```python
from build123d import *

# Parameters (mm, degrees)
BOSS_EXTRUDE1_DEPTH = 4
CUT_EXTRUDE4_REACH  = 6
SKETCH2_R           = 1.55
CUT_EXTRUDE5_DEPTH  = 5
FILLET1_R           = 0.5


with BuildPart() as part:
    # Sketch1 → Boss-Extrude1 (new body)
    with BuildSketch(Plane.XY):
        with BuildLine():
            Line((-10, 14), (-7.553754025, 14))
            Line((-7.553754025, 14), (-7.550510257, 12.5))
            ThreePointArc((-7.550510257, 12.5), (-6.759629651, 8.677124344), (-10, 6.5))
            Line((-10, 6.5), (-11.5, 6.5))
            Line((-11.5, 6.5), (-11.5, -6.5))
            Line((-11.5, -6.5), (-10, -6.5))
            ThreePointArc((-10, -6.5), (-6.774250172, -8.641862287), (-7.496564289, -12.445978258))
            Line((-7.496564289, -12.445978258), (-7.493203699, -14))
            Line((-7.493203699, -14), (-10, -14))
            ThreePointArc((-10, -14), (-12.474873734, -12.974873734), (-13.5, -10.5))
            Line((-13.5, -10.5), (-13.5, 10.5))
            ThreePointArc((-13.5, 10.5), (-12.474873734, 12.974873734), (-10, 14))
        make_face()
    extrude(amount=BOSS_EXTRUDE1_DEPTH)

    # Sketch2 → Cut-Extrude4 (cut, up to next)
    with BuildSketch(Plane.XY, mode=Mode.PRIVATE) as cut_extrude4_sk1:
        with Locations((-10, -10)):
            Circle(SKETCH2_R)
    cut_extrude4_tool1 = extrude(cut_extrude4_sk1.sketch, amount=CUT_EXTRUDE4_REACH, mode=Mode.PRIVATE) & part.part
    add(cut_extrude4_tool1.solids().sort_by_distance((-10, -10, 0))[0], mode=Mode.SUBTRACT)
    # Sketch2 → Cut-Extrude4 (cut, up to next)
    with BuildSketch(Plane.XY, mode=Mode.PRIVATE) as cut_extrude4_sk2:
        with Locations((-10, 10)):
            Circle(SKETCH2_R)
    cut_extrude4_tool2 = extrude(cut_extrude4_sk2.sketch, amount=CUT_EXTRUDE4_REACH, mode=Mode.PRIVATE) & part.part
    add(cut_extrude4_tool2.solids().sort_by_distance((-10, 10, 0))[0], mode=Mode.SUBTRACT)

    # Sketch3 → Cut-Extrude5 (cut, through all)
    with BuildSketch(Plane.XY.offset(4)):
        with BuildLine():
            Line((-9.034256252, 11.212369174), (-6.716684452, 11.212369174))
            ThreePointArc((-6.716684452, 11.212369174), (-6.5, 10), (-6.716684452, 8.787630826))
            Line((-6.716684452, 8.787630826), (-9.034256252, 8.787630826))
            ThreePointArc((-9.034256252, 8.787630826), (-8.45, 10), (-9.034256252, 11.212369174))
        make_face()
    cut_extrude5 = extrude(amount=-CUT_EXTRUDE5_DEPTH, mode=Mode.SUBTRACT)

    # Mirror1: Cut-Extrude5 across plane
    add(cut_extrude5.mirror(Plane(origin=(0, 0, 0), x_dir=(0, 0, 1), z_dir=(0, -1, 0))), mode=Mode.SUBTRACT)

    # Fillet1
    fillet1_edges = [part.edges().sort_by_distance(p)[0] for p in [
        (-6.716684452, 11.212369174, 2),
        (-6.716684452, 8.787630826, 2),
        (-6.716684452, -8.787630826, 2),
        (-6.716684452, -11.212369174, 2),
    ]]
    fillet(fillet1_edges, radius=FILLET1_R)


solid = part.part
```
Geometry check sheet. Reference: the model listing, model coordinates, mm. A direction names the side the tool comes from. Give positions to 0.01 mm unless a question says otherwise; leave off trailing zeros. Order: outer loops, then holes, each group sorted by start corner. A loop starts at its lowest first (then second) coordinate and runs counter-clockwise, first axis right, second up. Notation, with made-up numbers: (16.25, -36) - (25.25, -36) arc R27 cw to (25.25, -9) - close; hole circle Ø1 at (35.5, 31). An arc over 180 degrees is marked (long way). Answer in a Markdown table with one row per item. Add a question column.
Q1. Cross-section at C-C, the plane y = -10. Enter the section's corners in (x, z), then the cut area to 3 significant figures.
Q2. Gauge pin test, flat ends, axial feed: pin 1 (2 mm diameter, centred on y = -1, z = 3, fed in from +X); pin 2 (0.8 mm diameter, centred on x = -11, z = 2.5, fed in from +Y). Record the tip position at first contact, or that the pin passes through.
Q3. Material ranges on probe 1 along Y at (x, z) = (-10, 1); probe 2 along Y at (x, z) = (-9.25, 2.1); probe 3 along X at (y, z) = (3.5, 0.3), recorded low to high. Write a range as from..to.
Q4. Cross-section at A-A, the plane z = 1.45. Enter the section's corners in (x, y).
Q5. Cross-section at B-B, the plane x = -9.5. Enter the section's corners in (y, z).
Q6. Tool access check on faces 1 (the flat face through (-11, -6.5, 2)), 2 (the flat face through (-12, 0, 4)). Record the directions out of +Z, -Z, +X, -X, +Y, -Y that give a thin tool (end or side, any length) a straight path to the whole face; none if there is none.
Q7. Cross-section at D-D, the plane x = -11. Enter the section's corners in (y, z), then the cut area to 3 significant figures.
Q8. Mould release check, pull along X, two halves, no side actions. Record for faces 3 (the cylindrical face through (-11.55, 10.05, 1.97)), 4 (the flat face through (-13.5, 0, 2)), 5 (the flat face through (-8, -8.788, 2)): pulls with the +X half, pulls with the -X half, needs draft (parallel to the pull), parting line crosses it, or undercut.
Check values:
| question | item | result |
|---|---|---|
| 1 | outline | (-13.5, 0) - (-11.55, 0) - (-11.55, 4) - (-13.5, 4) - close |
| 1 | area | 7.80 mm^2 |
| 2 | pin 1 | stops at x = -11.5 |
| 2 | pin 2 | stops at y = 13.95 |
| 3 | probe 1 | y = -14..-11.55, -8.45..-6.5, 6.5..8.45, 11.55..14 |
| 3 | probe 2 | y = -14..-11.36, -8.64..-6.58, 6.58..8.64, 11.36..14 |
| 3 | probe 3 | x = -13.5..-11.5 |
| 4 | outline | (-13.5, -10.5) arc R3.5 ccw to (-10, -14) - (-7.49, -14) - (-7.5, -12.45) arc R3.5 ccw to (-7.13, -12) arc R0.5 ccw to (-7.54, -11.21) - (-9.03, -11.21) arc R1.55 cw (long way) to (-9.03, -8.79) - (-7.54, -8.79) arc R0.5 ccw to (-7.13, -8) arc R3.5 ccw to (-10, -6.5) - (-11.5, -6.5) - (-11.5, 6.5) - (-10, 6.5) arc R3.5 ccw to (-7.13, 8) arc R0.5 ccw to (-7.54, 8.79) - (-9.03, 8.79) arc R1.55 cw (long way) to (-9.03, 11.21) - (-7.54, 11.21) arc R0.5 ccw to (-7.13, 12) arc R3.5 ccw to (-7.55, 12.5) - (-7.55, 14) - (-10, 14) arc R3.5 ccw to (-13.5, 10.5) - close |
| 5 | outline | (-14, 0) - (-11.47, 0) - (-11.47, 4) - (-14, 4) - close; (-8.53, 0) - (-6.54, 0) - (-6.54, 4) - (-8.53, 4) - close; (6.54, 0) - (8.53, 0) - (8.53, 4) - (6.54, 4) - close; (11.47, 0) - (14, 0) - (14, 4) - (11.47, 4) - close |
| 6 | face 1 | +Z, -Z, +X |
| 6 | face 2 | +Z, +X, -X, +Y, -Y |
| 7 | outline | (-13.85, 0) - (-11.18, 0) - (-11.18, 4) - (-13.85, 4) - close; (-8.82, 0) - (-6.5, 0) - (-6.5, 4) - (-8.82, 4) - close; (6.5, 0) - (8.82, 0) - (8.82, 4) - (6.5, 4) - close; (11.18, 0) - (13.85, 0) - (13.85, 4) - (11.18, 4) - close |
| 7 | area | 39.9 mm^2 |
| 8 | face 3 | undercut |
| 8 | face 4 | pulls with the -X half |
| 8 | face 5 | needs draft |
